Can you work these out from the model? Positions are in its coordinate system, mm. Face numbers are marked on the shaded views. A direction names the side the tool comes from. Give positions to 0.01 mm unless a question says otherwise; leave off trailing zeros. Write each loop counter-clockwise with the first axis right and the second up, starting at its lowest first coordinate (ties: lowest second). Pieces come first, ordered by that corner, then holes.
1. Suppose I cut it at C-C (z = 8.5). Please give me the cut outline in (x, y).
2. Suppose I cut it at A-A (x = 3). Please give me the cut outline in (y, z).
3. Suppose I cut it at B-B (y = 0). Please give me the cut outline in (x, z), and give its area (3 significant figures).
4. I'm going to push flat-ended pins straight in: pin 1 (2 mm diameter, centred on x = 23, y = 4, fed in from +Z); pin 2 (2 mm diameter, centred on x = 23.5, y = 1.5, fed in from -Z); pin 3 (3 mm diameter, centred on x = -13.5, y = -6, fed in from +Z). Where does each tip first touch, or does it pass through?
5. If I drill on probe 1 along X at (y, z) = (-3.5, 20); probe 2 along Z at (x, y) = (-5, 6.5); probe 3 along Z at (x, y) = (-22, -6.5), over which ranges is the centre line in solid material (lowest first)?
6. Suppose I cut it at D-D (x = 21). Please give me the cut outline in (y, z).
7. On a 3-axis mill with a long thin cutter (end or side, diameter ignored), from which of +Z, -Z, +X, -X, +Y, -Y can I reach the whole of each face in a straight line? I mean the marked faces 1, 2, 3, 4 and 5. Say none if no direction works.
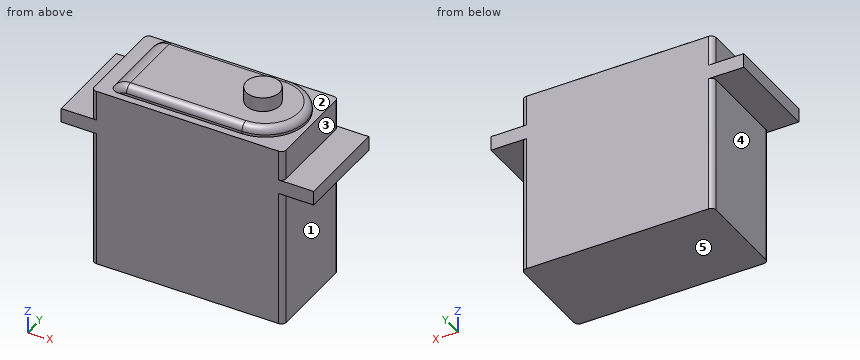
```python
from build123d import *

# Parameters (mm, degrees)
SKETCH1_W           = 40.132
SKETCH1_H           = 20.066
BOSS_EXTRUDE1_DEPTH = 38.1
SKETCH2_W           = 6.35
SKETCH2_H           = 20.066
BOSS_EXTRUDE2_DEPTH = 3
BOSS_EXTRUDE4_DEPTH = 2
SKETCH5_R           = 3.5
BOSS_EXTRUDE3_DEPTH = 3
FILLET2_R           = 4
FILLET3_R           = 1.5
FILLET4_R           = 1


with BuildPart() as part:
    # Sketch1 → Boss-Extrude1 (new body)
    with BuildSketch(Plane.XY):
        Rectangle(SKETCH1_W, SKETCH1_H)
    extrude(amount=BOSS_EXTRUDE1_DEPTH)

    # Sketch2 → Boss-Extrude2 (add)
    with BuildSketch(Plane(origin=(0, 0, 31.75), x_dir=(-1, 0, 0), z_dir=(0, 0, -1))):
        with Locations((23.241, 0)):
            Rectangle(SKETCH2_W, SKETCH2_H)
        with Locations((-23.241, 0)):
            Rectangle(SKETCH2_W, SKETCH2_H)
    extrude(amount=BOSS_EXTRUDE2_DEPTH)

    # Sketch6 → Boss-Extrude4 (add)
    with BuildSketch(Plane.XY.offset(38.1)):
        with BuildLine():
            Line((-17.066, 8.533), (10.533, 8.533))
            ThreePointArc((10.533, 8.533), (19.066, 0), (10.533, -8.533))
            Line((10.533, -8.533), (-17.066, -8.533))
            Line((-17.066, -8.533), (-17.066, 8.533))
        make_face()
    extrude(amount=BOSS_EXTRUDE4_DEPTH)

    # Sketch5 → Boss-Extrude3 (add)
    with BuildSketch(Plane.XY.offset(40.1)):
        with Locations((10.033, 0)):
            Circle(SKETCH5_R)
    extrude(amount=BOSS_EXTRUDE3_DEPTH)

    # Fillet2
    # the kernel refuses this fillet: 4 mm, written as the material it takes off along each edge
    with BuildSketch(Plane(origin=(-17.066, -17.193254038, 40.1), x_dir=(0, 0, -1), z_dir=(0, 1, 0))) as fillet2_piece_1:
        with BuildLine():
            CenterArc((4, -3.464101615), FILLET2_R, 120, 60)
            Line((0, -3.464101615), (-0.08, -3.464101615))
            Line((-0.08, -3.464101615), (-0.08, 0))
            Line((-0.08, 0), (0, 0.08))
            ThreePointArc((0, 0.08), (1, 0.08), (1.96, 0.069282032))
            Line((1.96, 0.069282032), (2, 0))
        make_face()
    extrude(amount=34.386508076, mode=Mode.SUBTRACT)

    # Fillet3
    fillet3_edges = [part.edges().sort_by_distance(p)[0] for p in [
        (19.066, 0, 40.1),
        (-1.534449192, 8.533, 40.1),
        (-1.534449192, -8.533, 40.1),
        (-15.601898385, -8.533, 39.564101615),
        (-15.601898385, 8.533, 39.564101615),
    ]]
    fillet(fillet3_edges, radius=FILLET3_R)

    # Fillet4
    fillet4_edges = [part.edges().sort_by_distance(p)[0] for p in [
        (-20.066, -10.033, 14.375),
        (-20.066, 10.033, 14.375),
        (20.066, 10.033, 14.375),
        (20.066, -10.033, 14.375),
        (20.066, -10.033, 34.925),
        (-20.066, -10.033, 34.925),
        (-20.066, 10.033, 34.925),
        (20.066, 10.033, 34.925),
    ]]
    fillet(fillet4_edges, radius=FILLET4_R)


solid = part.part
```
Checks:
1. outline: (-20.07, -9.03) arc R1 ccw to (-19.07, -10.03) - (19.07, -10.03) arc R1 ccw to (20.07, -9.03) - (20.07, 9.03) arc R1 ccw to (19.07, 10.03) - (-19.07, 10.03) arc R1 ccw to (-20.07, 9.03) - close
2. outline: (-10.03, 0) - (10.03, 0) - (10.03, 38.1) - (8.53, 38.1) - (8.53, 38.6) arc R1.5 ccw to (7.03, 40.1) - (-7.03, 40.1) arc R1.5 ccw to (-8.53, 38.6) - (-8.53, 38.1) - (-10.03, 38.1) - close
3. outline: (-26.42, 28.75) - (-20.07, 28.75) - (-20.07, 0) - (20.07, 0) - (20.07, 28.75) - (26.42, 28.75) - (26.42, 31.75) - (20.07, 31.75) - (20.07, 38.1) - (19.07, 38.1) - (19.07, 38.6) arc R1.5 ccw to (17.57, 40.1) - (13.53, 40.1) - (13.53, 43.1) - (6.53, 43.1) - (6.53, 40.1) - (-13.6, 40.1) arc R4 ccw to (-17.07, 38.1) - (-20.07, 38.1) - (-20.07, 31.75) - (-26.42, 31.75) - close
3. area: 1,660 mm2
4. pin 1: stops at z = 31.75
4. pin 2: stops at z = 28.75
4. pin 3: stops at z = 40.1
5. probe 1: x = -20.07 to 20.07
5. probe 2: z = 0 to 40.1
5. probe 3: z = 28.75 to 31.75
6. outline: (-10.03, 28.75) - (10.03, 28.75) - (10.03, 31.75) - (-10.03, 31.75) - close
7. face 1: -Z, +X, +Y, -Y
7. face 2: +Z
7. face 3: +Z, +X, +Y, -Y
7. face 4: -Z, -X, +Y, -Y
7. face 5: -Z, +X, -X, +Y, -Y
